from build123d import *

# Parameters (mm, degrees)
BOSS_EXTRUDE1_DEPTH   = 3
BOSS_EXTRUDE1_2_DEPTH = 3
BOSS_EXTRUDE1_3_DEPTH = 3
BOSS_EXTRUDE1_4_DEPTH = 3
BOSS_EXTRUDE1_5_DEPTH = 3
BOSS_EXTRUDE1_6_DEPTH = 3
BOSS_EXTRUDE2_DEPTH   = 3
BOSS_EXTRUDE3_DEPTH   = 4
BOSS_EXTRUDE4_DEPTH   = 5
BOSS_EXTRUDE5_DEPTH   = 2.5
SKETCH7_R             = 8.625
BOSS_EXTRUDE6_DEPTH   = 10
FILLET1_R             = 1


with BuildPart() as part:
    # Sketch1 → Boss-Extrude1 (new body)
    with BuildSketch(Plane.XY):
        Polygon((-157.708306786, 40.356035083), (-152.304819575, 44.329897546), (-149.391723249, 22.316986717), (-150.505818609, 20.162863795), (-151.029240558, 19.996298037), (-154.910321184, 19.21296233), align=None)
    extrude(amount=-BOSS_EXTRUDE1_DEPTH)



with BuildPart() as body_2:
    # Sketch1 → Boss-Extrude1 2 (new body)
    with BuildSketch(Plane.XY):
        Polygon((-143.200182369, 23.681067988), (-141.771708727, 22.942272705), (-141.417062609, 23.055129835), (-128.353286026, 23.842538892), (-126.923061182, 25.367546815), (-126.299118711, 45.160018639), (-145.963883673, 45.026358385), align=None)
    extrude(amount=-BOSS_EXTRUDE1_2_DEPTH)


with BuildPart() as body_3:
    # Sketch1 → Boss-Extrude1 3 (new body)
    with BuildSketch(Plane.XY):
        Polygon((-107.452313856, 22.751941247), (-105.8273555, 24.022922299), (-102.964187331, 40.958018331), (-119.948602388, 43.563327727), (-120.531202342, 25.369443818), (-119.203583194, 24.12433954), (-118.788909935, 24.137639341), align=None)
    extrude(amount=-BOSS_EXTRUDE1_3_DEPTH)


with BuildPart() as body_4:
    # Sketch1 → Boss-Extrude1 4 (new body)
    with BuildSketch(Plane.XY):
        Polygon((-99.567663538, 22.722793004), (-98.442870148, 21.001338348), (-89.386000699, 19.102739522), (-87.194407263, 27.543337474), (-96.584441251, 40.806132568), align=None)
    extrude(amount=-BOSS_EXTRUDE1_4_DEPTH)


with BuildPart() as body_5:
    # Sketch1 → Boss-Extrude1 5 (new body)
    with BuildSketch(Plane.XY):
        Polygon((-129.565242632, 10.790123413), (-130.675013398, 17.075689336), (-130.720095352, 18.270412872), (-128.136441147, 18.426140636), (-119.436419139, 18.705176142), (-106.720361509, 17.114886687), (-106.498771051, 15.1412078), (-109.869761523, 10.324632035), (-125.066433071, 7.64152887), align=None)
    extrude(amount=-BOSS_EXTRUDE1_5_DEPTH)


with BuildPart() as body_6:
    # Sketch1 → Boss-Extrude1 6 (new body)
    with BuildSketch(Plane.XY):
        Polygon((-105.107164744, 5.681988451), (-98.463483991, -31.946767529), (-120.749282124, -35.881517012), (-127.392962877, 1.747238969), align=None)
    extrude(amount=-BOSS_EXTRUDE1_6_DEPTH)


with BuildPart() as part_1:
    add(part.part)

    add(body_2.part)  # Boss-Extrude2 merges body 2

    add(body_3.part)  # Boss-Extrude2 merges body 3

    add(body_4.part)  # Boss-Extrude2 merges body 4

    add(body_5.part)  # Boss-Extrude2 merges body 5

    add(body_6.part)  # Boss-Extrude2 merges body 6
    # Sketch2 → Boss-Extrude2 (add)
    with BuildSketch(Plane.XY):
        Polygon((-154.778828939, 18.219336743), (-149.003710401, 19.384954517), (-148.676438789, 16.911915522), (-130.758309274, 19.283125657), (-130.675013398, 17.075689336), (-129.565242632, 10.790123413), (-127.392962877, 1.747238969), (-120.749282124, -35.881517012), (-98.463483991, -31.946767529), (-105.107164744, 5.681988451), (-106.498771051, 15.1412078), (-106.720361509, 17.114886687), (-89.640117023, 13.5343413), (-89.386000699, 19.102739522), (-87.194407263, 27.543337474), (-96.584441251, 40.806132568), (-102.964187331, 40.958018331), (-119.948602388, 43.563327727), (-126.299118711, 45.160018639), (-145.963883673, 45.026358385), (-152.304819575, 44.329897546), (-157.708306786, 40.356035083), align=None)
    extrude(amount=BOSS_EXTRUDE2_DEPTH)

    # Sketch3 → Boss-Extrude3 (add)
    with BuildSketch(Plane(origin=(0, 0, -3), x_dir=(-1, 0, 0), z_dir=(0, 0, -1))):
        Polygon((119.436419139, 18.705176142), (130.720095352, 18.270412872), (130.675013398, 17.075689336), (129.565242632, 10.790123413), (125.066433071, 7.64152887), (109.869761523, 10.324632035), (106.498771051, 15.1412078), (106.720361509, 17.114886687), align=None)
    extrude(amount=BOSS_EXTRUDE3_DEPTH)

    # Sketch4 → Boss-Extrude4 (add)
    with BuildSketch(Plane(origin=(0, 0, -3), x_dir=(-1, 0, 0), z_dir=(0, 0, -1))):
        Polygon((105.107164744, 5.681988451), (127.392962877, 1.747238969), (120.749282124, -35.881517012), (98.463483991, -31.946767529), align=None)
    extrude(amount=BOSS_EXTRUDE4_DEPTH)

    # Sketch5 → Boss-Extrude5 (add)
    with BuildSketch(Plane(origin=(0, 0, 0), x_dir=(-1, 0, 0), z_dir=(0, 0, -1))):
        Polygon((106.498771051, 15.1412078), (105.107164744, 5.681988451), (127.392962877, 1.747238969), (129.565242632, 10.790123413), (125.066433071, 7.64152887), (109.869761523, 10.324632035), align=None)
    extrude(amount=BOSS_EXTRUDE5_DEPTH)

    # Sketch7 → Boss-Extrude6 (add)
    with BuildSketch(Plane.XY.offset(3)):
        with Locations((-108.375015851, 26.614118497)):
            Circle(SKETCH7_R)
    extrude(amount=BOSS_EXTRUDE6_DEPTH)

    # Fillet1
    fillet1_edges = [part_1.edges().sort_by_distance(p)[0] for p in [
        (-117.000015851, 26.614118497, 3),
    ]]
    fillet(fillet1_edges, radius=FILLET1_R)


solid = part_1.part
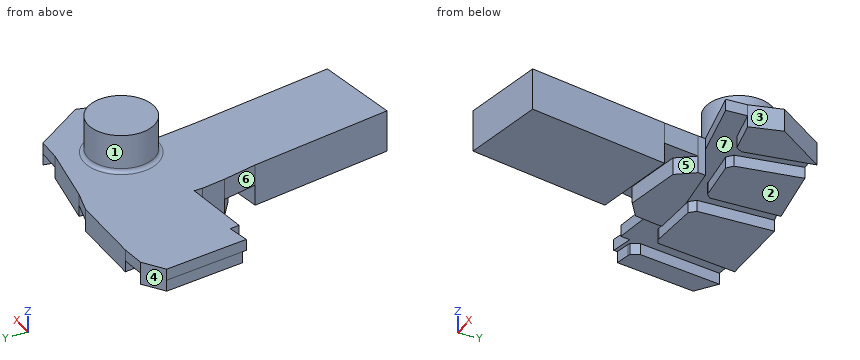
Can you work these out from the model? Positions are in its coordinate system, mm. Face numbers are marked on the shaded views. A direction names the side the tool comes from. Give positions to 0.01 mm unless a question says otherwise; leave off trailing zeros. Order: outer loops, then holes, each group sorted by start corner. A loop starts at its lowest first (then second) coordinate and runs counter-clockwise, first axis right, second up. Notation, with made-up numbers: M 15,-11 L 33,-11 A25 cw 33,24 Z; hole C 73,-4.5 d3. An arc over 180 degrees is marked long. Use one line per item in the form item = value. Start each with the question number.
Item 1: If we section it at C-C (x = -138): Write out the boundary of the cut face in (y, z).
Item 2: If we section it at D-D (y = 3): Write out the boundary of the cut face in (x, z), then the cut area to 3 significant figures.
Item 3: If I drill on line 1 along X through (y, z) = (27.5, -1); line 2 along Z through (x, y) = (-145.5, 22); line 3 along Z through (x, y) = (-112, 31.5), over which ranges is the centre line in solid material (lowest first)?
Item 4: If we section it at B-B (z = -1.5): State how many separate pieces and enclosed holes the cut face has, then the cut area to 3 significant figures.
Item 5: Will these pins go through, and if not, where does the flat tip stop? pin 1 Ø5.5 at (x, y) = (-115.5, 37) entering from -Z; pin 2 Ø3 at (x, z) = (-150.5, 2.5) entering from -Y; pin 3 Ø4 at (y, z) = (27, 6.5) entering from +X.
Item 6: We'd pull the mould along X, two halves only. Please class the marked faces 5, 6 and 7: +X half, -X half, draft (parallel to the pull), parting line (faces both ways), or undercut.
Item 7: If we section it at A-A (z = -6): Write out the boundary of the cut face in (x, y), then the cut area to 3 significant figures.
Item 8: For the marked faces 1, 2, 3 and 4, which set-ups out of +Z, -Z, +X, -X, +Y, -Y let a thin tool reach every point of the face, with its end or its side?
Outcome:
q1.outline = M 18.32,0 L 23.26,0 L 23.26,-3 L 45.08,-3 L 45.08,3 L 18.32,3 Z
q2.outline = M -127.69,-2.5 L -120.3,-2.5 L -120.3,-8 L -104.63,-8 L -104.63,3 L -127.69,3 Z
q2.area = 213 mm2
q3.line_1 = -156.01 to -150.08, -143.69 to -126.86, -120.46 to -105.24, -98.78 to -87.21
q3.line_2 = 0 to 3
q3.line_3 = -3 to 13
q4.separate_pieces = 5
q4.enclosed_holes = 0
q4.area = 2,180 mm2
q5.pin_1 = -3
q5.pin_2 = 18.78
q5.pin_3 = -99.75
q6.face_5 = +X half
q6.face_6 = -X half
q6.face_7 = undercut
q7.outline = M -130.72,18.27 L -130.68,17.08 L -129.57,10.79 L -125.07,7.64 L -109.87,10.32 L -106.5,15.14 L -106.72,17.11 L -119.44,18.71 Z; M -127.39,1.75 L -120.75,-35.88 L -98.46,-31.95 L -105.11,5.68 Z
q7.area = 1,070 mm2
q8.face_1 = +Z
q8.face_2 = -Z, +X, -X, +Y
q8.face_3 = +Z, -Z, +X, -Y
q8.face_4 = +Z, -Z, -X, +Y
